Autodesk Inventor part; units mm, degrees
ref_plane "YZ Plane" through (0, 0, 0) normal (1, 0, 0) x (0, 1, 0)
ref_plane "XZ Plane" through (0, 0, 0) normal (0, 1, 0) x (-1, 0, 0)
ref_plane "XY Plane" through (0, 0, 0) normal (0, 0, 1) x (1, 0, 0)
sketch "Esboço1" plane through (0, 0, 0) normal (0, 0, 1) x (1, 0, 0)
  line L0 (-100, 5) -> (100, 5)
  line L1 (100, 5) -> (100, -5)
  line L2 (100, -5) -> (-100, -5)
  line L3 (-100, -5) -> (-100, 5)
  line L4 (-100, 5) -> (100, -5) construction
  line L5 (100, 5) -> (-100, -5) construction
  point P0 (0, 0)
  dimension "d0" = 200
  dimension "d1" = 10
extrude "Extrusão1" add sketch "Esboço1" along normal blind 100
sketch "Esboço2" plane through (0, 0, 100) normal (0, 0, 1) x (1, 0, 0)
  line L0 (100, 5) -> (-100, 5)
  line L1 (100, 5) -> (-100, 5)
  line L2 (-100, -5) -> (100, -5)
  line L3 (0, -5) -> (0, 195) construction
  line L4 (0, 195) -> (-100, 5)
  line L5 (0, 195) -> (100, 5)
  point P0 (0, 0)
  point P1 (0, 5)
  dimension "d20" = 200
extrude "Extrusão2" add sketch "Esboço2" against normal blind 15
sketch "Esboço3" plane through (0, 0, 0) normal (0, 0, -1) x (-1, 0, 0)
  line L0 (-100, 5) -> (100, 5)
  line L1 (100, -5) -> (-100, -5)
  line L2 (0, -5) -> (0, 195) construction
  line L3 (-100, -5) -> (-100, 5)
  line L4 (0, 195) -> (-100, 5)
  line L5 (0, 195) -> (100, 5)
  point P0 (0, 0)
  dimension "d21" = 200
extrude "Extrusão3" add sketch "Esboço3" against normal blind 15
sketch "Esboço4" plane through (0, 0, 100) normal (0, 0, 1) x (1, 0, 0)
  circle A0 centre (0, 155) radius 4.25
  line L0 (-100, -5) -> (100, -5)
  line L1 (100, 5) -> (0, 195)
  line L2 (0, 195) -> (0, -5) construction
  point P0 (0, 0)
  dimension "d13" = 8.5
  dimension "d22" = 160
extrude "Extrusão4" cut sketch "Esboço4" against normal through all
fillet "Arredondamento3" radius 10 2 edges at (0, 195, 92.5) (0, 195, 7.5)
sketch "Esboço5" plane through (0, 0, 100) normal (0, 0, 1) x (1, 0, 0)
  circle A0 centre (0, 155) radius 4.25
  circle A1 centre (0, 155) radius 10.975
  point P0 (0, 0)
  dimension "d25" = 21.95
extrude "Extrusão5" cut sketch "Esboço5" against normal blind 7
sketch "Esboço6" plane through (0, 0, 0) normal (0, 0, -1) x (-1, 0, 0)
  circle A0 centre (0, 155) radius 4.25
  circle A1 centre (0, 155) radius 10.975
  point P0 (0, 0)
  dimension "d28" = 21.95
extrude "Extrusão6" cut sketch "Esboço6" against normal blind 7
sketch "Esboço7" plane through (0, 0, 0) normal (0, 0, -1) x (-1, 0, 0)
  circle A0 centre (0, 155) radius 10.975
  circle A1 centre (0, 155) radius 18.6299
  line L0 (100, 5) -> (8.8492, 178.1866)
  line L1 (15.3264, 144.4089) -> (88.6995, 5)
  line L2 (100, 5) -> (-100, 5)
  line L3 (88.6995, 5) -> (-88.6995, 5)
  line L4 (-15.3264, 144.4089) -> (-88.6995, 5)
  line L5 (100, 5) -> (8.8492, 178.1866)
  line L6 (-8.8492, 178.1866) -> (-100, 5)
  circle A2 centre (0, 155) radius 4.25
  line L7 (0, 155) -> (0, -5.3042)
  line L8 (10, 139.2815) -> (10, 5)
  line L9 (-10, 139.2815) -> (-10, 5)
  point P0 (0, 0)
  point P1 (-10.946, 174.2026)
  point P2 (10.946, 174.2026)
  dimension "d31" = 10
  dimension "d32" = 10
  dimension "d39" = 10
  dimension "d40" = 10
extrude "Extrusão7" cut sketch "Esboço7" against normal through all contours L9 L2 L4 A1 | A1 L1 L2 L8
chamfer "Chanfro1" distance 5 angle 45 8 edges at (-10, 139.2815, 92.5) (10, 139.2815, 92.5) (10, 139.2815, 7.5) (-10, 139.2815, 7.5) (10, 5, 7.5) (-10, 5, 7.5) (-10, 5, 92.5) (10, 5, 92.5)
fillet "Arredondamento5" radius 2 4 edges at (88.6995, 5, 92.5) (-88.6995, 5, 92.5) (88.6995, 5, 7.5) (-88.6995, 5, 7.5)
fillet "Arredondamento6" radius 10 2 edges at (-100, 5, 50) (100, 5, 50)
fillet "Arredondamento7" radius 10 4 edges at (100, 5, 92.5) (100, 5, 7.5) (-100, 5, 92.5) (-100, 5, 7.5)
properties part number "EncaixeBase"
The model under review builds one solid part; all positions refer to its coordinate system, in mm. A direction names the side the tool comes from. Round coordinates to 2 decimals unless told otherwise and drop trailing zeros. Write each loop counter-clockwise with the first axis right and the second up, starting at its lowest first coordinate (ties: lowest second). Pieces come first, ordered by that corner, then holes. Notation, with made-up numbers: M -0.5,23.25 L 16.5,23.25 A12 cw 16.5,42.25 Z; hole C 13.25,-31.75 d4. An arc over 180 degrees is marked long. Answer as CSV lines item,"result". Start each with the question number.
Q1. Clearance check with flat-ended pins moving along their axes: P1, Ø11, axis at x = 2, y = 150, coming from the -Z side; P2, Ø7.5, axis at y = 79.5, z = 89, coming from the +X side; P3, Ø7.5, axis at x = 0, y = 155, coming from the +Z side; P4, Ø12, axis at x = 11, z = 52.5, coming from the +Y side. State where each tip first meets the part, or that it passes through.
Q2. The part is to be moulded in two halves that separate along Y. For faces 1 (the face through (97.15, 1.99, 50.49)), 2 (the face through (1, -5, 49)), 3 (the face through (-10, 73, 92)), say which applies: +Y half, -Y half, draft (parallel to the pull), parting line (faces both ways), or undercut.
Q3. Wall thickness on line 1 along Y through (x, z) = (0, 13.25); line 2 along Y through (x, z) = (0, 94.75) (3 decimals); line 3 along Z through (x, y) = (5, 17): over which ranges is each line inside the solid? List them lowest first.
Q4. Tool access review of faces 4 (the face through (-12, 8, 7)), 5 (the face through (1.43, 165.88, 3.45)), 6 (the face through (-96.99, 2.15, 50.49)): name each direction out of +Z, -Z, +X, -X, +Y, -Y from which nothing blocks a thin tool from reaching the whole face with its end or side.
Q5. Consider section D-D, the plane z = 10. Give the boundary of the cut face in (x, y).
Q6. Consider section B-B, the plane y = 124. Give the boundary of the cut face in (x, z), then the cut area to 3 significant figures.
Q7. Consider section C-C, the plane y = 155. Give the boundary of the cut face in (x, z) (3 decimals).
Q8. Consider section A-A, the plane x = 0. Give the boundary of the cut face in (y, z) (3 decimals).
Result set:
1,P1,"stops at z = 7"
1,P2,"stops at x = 62.76"
1,P3,"passes through"
1,P4,"stops at y = 5"
2,face 1,"+Y half"
2,face 2,"-Y half"
2,face 3,"undercut"
3,line 1,"y = -5 to 150.75, 159.25 to 183.53"
3,line 2,"y = -5 to 144.025, 165.975 to 183.529"
3,line 3,"z = 0 to 15, 85 to 100"
4,face 4,"+Z, -Z"
4,face 5,"-Z"
4,face 6,"-X, +Y"
5,outline,"M -100,-5 L 100,-5 L 100,2.53 A10 ccw 98.85,7.19 L 8.85,178.19 A10 ccw -8.85,178.19 L -98.85,7.19 A10 ccw -100,2.53 Z; hole M -87.16,7.93 A2 ccw -85.39,5 L -15,5 L -10,10 L -10,134.28 L -13.82,142.51 A18.63 cw -15.33,144.41 Z; hole C 0,155 d8.5; hole M 10,10 L 15,5 L 85.39,5 A2 ccw 87.16,7.93 L 15.33,144.41 A18.63 cw 13.82,142.51 L 10,134.28 Z"
6,outline,"M -37.37,0 L -26.07,0 L -26.07,15 L -37.37,15 Z; M -37.37,85 L -26.07,85 L -26.07,100 L -37.37,100 Z; M -10,0 L 10,0 L 10,15 L -10,15 Z; M -10,85 L 10,85 L 10,100 L -10,100 Z; M 26.07,0 L 37.37,0 L 37.37,15 L 26.07,15 Z; M 26.07,85 L 37.37,85 L 37.37,100 L 26.07,100 Z"
6,area,"1,280 mm²"
7,outline,"M -21.053,0 L -10.975,0 L -10.975,7 L -4.25,7 L -4.25,15 L -21.053,15 Z; M -21.053,85 L -4.25,85 L -4.25,93 L -10.975,93 L -10.975,100 L -21.053,100 Z; M 4.25,7 L 10.975,7 L 10.975,0 L 21.053,0 L 21.053,15 L 4.25,15 Z; M 4.25,85 L 21.053,85 L 21.053,100 L 10.975,100 L 10.975,93 L 4.25,93 Z"
8,outline,"M -5,0 L 144.025,0 L 144.025,7 L 150.75,7 L 150.75,15 L 5,15 L 5,85 L 150.75,85 L 150.75,93 L 144.025,93 L 144.025,100 L -5,100 Z; M 159.25,7 L 165.975,7 L 165.975,0 L 183.529,0 L 183.529,15 L 159.25,15 Z; M 159.25,85 L 183.529,85 L 183.529,100 L 165.975,100 L 165.975,93 L 159.25,93 Z"
